Input: part model. Units: mm. Frame: model coordinates. Face numbers are marked on the shaded views. A direction names the side the tool comes from. Round coordinates to 2 decimals unless told otherwise and drop trailing zeros. Loops run counter-clockwise (first coordinate to the right, second up) from the corner with the lowest first, then second, coordinate; pieces in that order, holes last.
1) Access query for the marked faces 1 and 2. Directions: +Z, -Z, +X, -X, +Y, -Y. A direction counts if a zero-diameter tool reaches every point of the face in a straight line with its end or side. Return the directions, or none.
2) First-contact query: pin 1 (1.7 mm diameter, centred on y = -4, z = 69, fed in from -X); pin 2 (2 mm diameter, centred on y = 2.5, z = 57, fed in from -X); pin 3 (2 mm diameter, centred on x = 1.5, y = -4.5, fed in from -Z); pin 4 (4 mm diameter, centred on x = -2.5, z = 85, fed in from -Y). Flat tips, straight axial feed; report the tip coordinate or a pass-through.
3) Section D-D, the plane z = 29. Return loops of the section in (x, y), and give its area (3 significant figures).
4) Section B-B, the plane z = 62.5. Return loops of the section in (x, y), and give its area (3 significant figures).
5) Ray query, line 1 along Z through (x, y) = (1.5, -5); line 2 along X through (y, z) = (0.25, 52); line 3 along X through (y, z) = (2.5, 47.5). Return the intervals inside material, ascending.
6) Section C-C, the plane x = 3.75. Return loops of the section in (y, z).
7) Section A-A, the plane y = 0. Return loops of the section in (x, z).
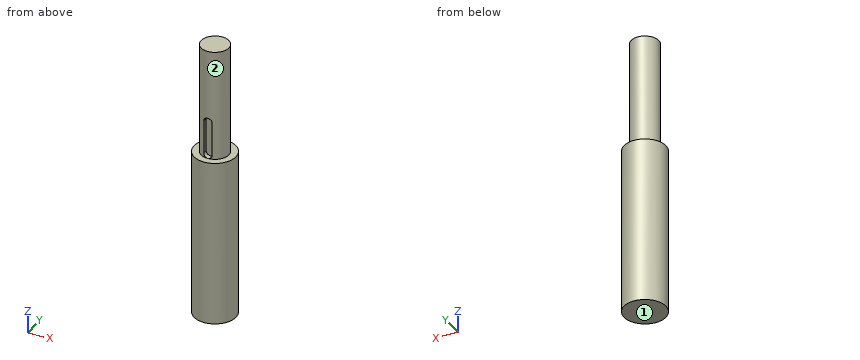
from build123d import *

# Parameters (mm, degrees)
SKETCH_1_R           = 7.5
EXTRUDE_1_DEPTH      = 100
SKETCH_2_OUTSIDE_W   = 37.446
SKETCH_2_OUTSIDE_H   = 37.446
SKETCH_2_OUTSIDE_R   = 5
CUT_EXTRUDE_1_DEPTH  = 40
CUT_EXTRUDE_START    = 5
CUT_EXTRUDE_13_DEPTH = 1.8


with BuildPart() as part:
    # 草图1 → 凸台-拉伸1 (new body)
    with BuildSketch(Plane.XY):
        Circle(SKETCH_1_R)
    extrude(amount=EXTRUDE_1_DEPTH)

    # 草图2 outside → 切除-拉伸1 (cut)
    with BuildSketch(Plane.XY.offset(100)):
        Rectangle(SKETCH_2_OUTSIDE_W, SKETCH_2_OUTSIDE_H)
        Circle(SKETCH_2_OUTSIDE_R, mode=Mode.SUBTRACT)
    extrude(amount=-CUT_EXTRUDE_1_DEPTH, mode=Mode.SUBTRACT)

    # 草图33 → 切除-拉伸13 (cut)
    with BuildSketch(Plane(origin=(-20, 0, 100), x_dir=(0, 0, 1), z_dir=(1.0206823934513925e-11, -1.0, 0)).offset(CUT_EXTRUDE_START)):
        with BuildLine():
            Line((-38.5, -18.5), (-26.5, -18.5))
            ThreePointArc((-26.5, -18.5), (-25, -20), (-26.5, -21.5))
            Line((-26.5, -21.5), (-38.5, -21.5))
            ThreePointArc((-38.5, -21.5), (-40, -20), (-38.5, -18.5))
        make_face()
    extrude(amount=-CUT_EXTRUDE_13_DEPTH, mode=Mode.SUBTRACT)


solid = part.part
Final values:
1. face 1: -Z, +X, -X, +Y, -Y
1. face 2: +Z
2. pin 1: stops at x = -3.88
2. pin 2: stops at x = -7.35
2. pin 3: stops at z = 0
2. pin 4: stops at y = -4.97
3. outline: circle Ø15 at (0, 0)
3. area: 177 mm2
4. outline: (-1.5, -4.77) - (-1.5, -3.2) - (1.5, -3.2) - (1.5, -4.77) arc R5 ccw (long way) to start
4. area: 73.4 mm2
5. line 1: z = 0 to 60
5. line 2: x = -7.5 to 7.5
5. line 3: x = -7.07 to 7.07
6. outline: (-6.5, 0) - (6.5, 0) - (6.5, 60) - (3.31, 60) - (3.31, 100) - (-3.31, 100) - (-3.31, 60) - (-6.5, 60) - close
7. outline: (-7.5, 0) - (7.5, 0) - (7.5, 60) - (5, 60) - (5, 100) - (-5, 100) - (-5, 60) - (-7.5, 60) - close
